```python
from build123d import *


with BuildPart() as part:
    # Sketch1 → Revolve2 (revolve)
    with BuildSketch(Plane.XY):
        Polygon((0, 34), (0, 26), (-1.2, 26), (-1.2, 28.5), (-2.2, 28.5), (-2.2, 28), (-5, 26), (-8, 26), (-12, 27), (-12, 28), (-8, 27), (-3, 30), (-8, 33), (-12, 32), (-12, 33), (-8, 34), (-5, 34), (-2.2, 32), (-2.2, 31.5), (-1.2, 31.5), (-1.2, 34), align=None)
    revolve(axis=Axis((-63.826580298, 0, 0), (1, 0, 0)))


solid = part.part
```
Design review of the part built by this model. Coordinates are the model's own, in mm. A direction names the side the tool comes from. Give positions to 0.01 mm unless a question says otherwise; leave off trailing zeros. Write each loop counter-clockwise with the first axis right and the second up, starting at its lowest first coordinate (ties: lowest second). Pieces come first, ordered by that corner, then holes.
(1) Wall thickness on line 1 along Y through (x, z) = (-8.25, 16.5); line 2 along Z through (x, y) = (-6.5, 21); line 3 along Y through (x, z) = (-3.25, 25): over which ranges is each line inside the solid? List them lowest first.
Checked values:
line 1: y = -29.66 to -28.51, -21.45 to -20.17, 20.17 to 21.45, 28.51 to 29.66
line 2: z = -26.74 to -24.28, -18.37 to -15.33, 15.33 to 18.37, 24.28 to 26.74
line 3: y = -21.16 to -16.85, -16.31 to -10.84, 10.84 to 16.31, 16.85 to 21.16
(2) Clearance check with flat-ended pins moving along their axes: pin 1 Ø3 at (x, z) = (-3, -5.5) entering from -Y; pin 2 Ø2 at (y, z) = (-12.5, -23.5) entering from -X; pin 3 Ø5 at (x, z) = (-8.5, -25) entering from +Y; pin 4 Ø3 at (x, y) = (-2, -18.5) entering from +Z. State where each tip first meets the part, or that it passes through.
Checked values:
pin 1: stops at y = -33.22
pin 2: stops at x = -12
pin 3: stops at y = 25.45
pin 4: stops at z = 29.31
(3) Mouldability with a two-part tool opening along X and no side actions: class faces 3 (the face through (-1.2, -23, -13)), 4 (the face through (-8.25, -5.65, -25.443)), 5 (the face through (-2.336, 30.615, 9.641)), 6 (the face through (-0.59, 18.28, 28.67)) as +X half, -X half, draft (parallel to the pull), parting line (faces both ways), or undercut.
Checked values:
face 3: undercut
face 4: -X half
face 5: undercut
face 6: draft
(4) Tool access review of faces 1 (the face through (-7.69, -5.89, -26.54)), 2 (the face through (-0.608, -20.633, -15.821)): name each direction out of +Z, -Z, +X, -X, +Y, -Y from which nothing blocks a thin tool from reaching the whole face with its end or side.
Checked values:
face 1: none
face 2: +X, -X
(5) Add section A-A (x = -10.5). Give the boundary of the cut face in (y, z) (3 decimals), and give its area (3 significant figures).
Checked values:
outline: circle Ø66.75 at (0, 0); circle Ø55.25 at (0, 0); hole circle Ø64.75 at (0, 0); hole circle Ø53.25 at (0, 0)
area: 377 mm2
